Design review of the part built by this model. Coordinates are the model's own, in mm. A direction names the side the tool comes from. Give positions to 0.01 mm unless a question says otherwise; leave off trailing zeros. Order: outer loops, then holes, each group sorted by start corner. A loop starts at its lowest first (then second) coordinate and runs counter-clockwise, first axis right, second up.
```python
from build123d import *

# Parameters (mm, degrees)
PAD_DEPTH    = 1
PAD001_DEPTH = 1
SKETCH002_W  = 3.5
SKETCH002_H  = 2
PAD002_DEPTH = 10
SKETCH003_R  = 2.5
POCKET_DEPTH = 2.001
SKETCH004_R  = 0.5
HOLE_DEPTH   = 10
HOLE_TIPS_R  = 0.5


with BuildPart() as part:
    # Sketch → Pad (new body)
    with BuildSketch(Plane.XY):
        with BuildLine():
            Line((-10, 5), (10, 5))
            Line((10, 5), (10, 1.5))
            ThreePointArc((10, -1.5), (11.5, 0), (10, 1.5))
            Line((10, -1.5), (10, -5))
            Line((10, -5), (-10, -5))
            Line((-10, -5), (-10, -1.5))
            ThreePointArc((-10, 1.5), (-11.5, 0), (-10, -1.5))
            Line((-10, 1.5), (-10, 5))
        make_face()
    extrude(amount=PAD_DEPTH)

    # Sketch001 (on Face10 of Pad) → Pad001 (join)
    with BuildSketch(Plane.XY.offset(1)):
        Polygon((-9, 4), (9, 4), (9, 0.489518), (7, 0.489518), (7, -0.510482), (9, -0.510482), (9, -4), (-9, -4), (-9, -0.49649), (-7, -0.49649), (-7, 0.50351), (-9, 0.50351), align=None)
    extrude(amount=PAD001_DEPTH)

    # Sketch002 (on Face23 of Pad001) → Pad002 (join)
    with BuildSketch(Plane.XY.offset(2)):
        with Locations((7.25, -3)):
            Rectangle(SKETCH002_W, SKETCH002_H)
        with Locations((7.25, 3)):
            Rectangle(SKETCH002_W, SKETCH002_H)
        with Locations((-7.25, 3)):
            Rectangle(SKETCH002_W, SKETCH002_H)
        with Locations((-7.25, -3)):
            Rectangle(SKETCH002_W, SKETCH002_H)
    extrude(amount=PAD002_DEPTH)

    # Sketch003 (on Face23 of Pad002) → Pocket (cut, through all)
    with BuildSketch(Plane.XY.offset(2)):
        Circle(SKETCH003_R)
    extrude(amount=-POCKET_DEPTH, mode=Mode.SUBTRACT)

    # Sketch004 (on Face42 of Pocket) → Hole (cut)
    with BuildSketch(Plane.XY.offset(12)):
        with Locations((8, -3)):
            Circle(SKETCH004_R)
        with Locations((-8, 3)):
            Circle(SKETCH004_R)
        with Locations((-8, -3)):
            Circle(SKETCH004_R)
        with Locations((8, 3)):
            Circle(SKETCH004_R)
    extrude(amount=-HOLE_DEPTH, mode=Mode.SUBTRACT)

    # Hole tips → Hole tip 1 section 0
    with BuildSketch(Plane.XY.offset(2), mode=Mode.PRIVATE) as hole_tip_1_s0:
        with Locations((8, -3)):
            Circle(HOLE_TIPS_R)
    loft([hole_tip_1_s0.sketch, Vertex(8, -3, 1.69957)], mode=Mode.SUBTRACT)

    # Hole tips → Hole tip 2 section 0
    with BuildSketch(Plane.XY.offset(2), mode=Mode.PRIVATE) as hole_tip_2_s0:
        with Locations((-8, 3)):
            Circle(HOLE_TIPS_R)
    loft([hole_tip_2_s0.sketch, Vertex(-8, 3, 1.69957)], mode=Mode.SUBTRACT)

    # Hole tips → Hole tip 3 section 0
    with BuildSketch(Plane.XY.offset(2), mode=Mode.PRIVATE) as hole_tip_3_s0:
        with Locations((-8, -3)):
            Circle(HOLE_TIPS_R)
    loft([hole_tip_3_s0.sketch, Vertex(-8, -3, 1.69957)], mode=Mode.SUBTRACT)

    # Hole tips → Hole tip 4 section 0
    with BuildSketch(Plane.XY.offset(2), mode=Mode.PRIVATE) as hole_tip_4_s0:
        with Locations((8, 3)):
            Circle(HOLE_TIPS_R)
    loft([hole_tip_4_s0.sketch, Vertex(8, 3, 1.69957)], mode=Mode.SUBTRACT)


solid = part.part
```
1. Machinability: for faces 5 (the face through (-10, -3.3, 0.5)), 6 (the face through (10, -3.2, 0.5)), 7 (the face through (-7, 2, 7)), 8 (the face through (-7, 0, 1.5)), which of the approach directions +Z, -Z, +X, -X, +Y, -Y give a long, thin tool a straight path to every point of the face, cutting with its end or side? Answer none if there is none.
Recorded:
face 5: +Z, -Z, -X, -Y
face 6: +Z, -Z, +X, -Y
face 7: +Z, +X, -X
face 8: +Z, -X
2. For pin 1 (6 mm diameter, centred on y = -3, z = 3, fed in from +X); pin 2 (1.1 mm diameter, centred on y = -4, z = 0.5, fed in from -X); pin 3 (1.6 mm diameter, centred on y = -3.5, z = 7, fed in from +X); pin 4 (4 mm diameter, centred on x = 0, y = 0, fed in from -Z), all flat-tipped, find the tip position at first contact; note any pin that passes through.
Recorded:
pin 1: stops at x = 11.29
pin 2: stops at x = -10
pin 3: stops at x = 9
pin 4: passes through
3. Draft analysis for pull direction X (two halves, no side actions). For faces 1 (the face through (-10, 3.2, 0.5)), 2 (the face through (8, -0.51, 1.5)), 3 (the face through (8.074, 2.969, 1.748)), 4 (the face through (8.074, -3.031, 1.748)), state which applies: pulls with the +X half, pulls with the -X half, needs draft (parallel to the pull), parting line crosses it, or undercut.
Recorded:
face 1: pulls with the -X half
face 2: needs draft
face 3: undercut
face 4: undercut
4. Take a section at B-B (x = 4.75). State the section outline as (y, z) points, then the cut area to 3 significant figures.
Recorded:
outline: (-5, 0) - (5, 0) - (5, 1) - (4, 1) - (4, 2) - (-4, 2) - (-4, 1) - (-5, 1) - close
area: 18.0 mm2
5. Take a section at A-A (z = 3). State the section outline as (x, y) points, then the cut area to 3 significant figures.
Recorded:
outline: (-9, -4) - (-5.5, -4) - (-5.5, -2) - (-9, -2) - close; (-9, 2) - (-5.5, 2) - (-5.5, 4) - (-9, 4) - close; (5.5, -4) - (9, -4) - (9, -2) - (5.5, -2) - close; (5.5, 2) - (9, 2) - (9, 4) - (5.5, 4) - close; hole circle Ø1 at (-8, -3); hole circle Ø1 at (-8, 3); hole circle Ø1 at (8, -3); hole circle Ø1 at (8, 3)
area: 24.9 mm2
6. Take a section at C-C (y = 0). State the section outline as (x, z) points, then the cut area to 3 significant figures.
Recorded:
outline: (-11.5, 0) - (-2.5, 0) - (-2.5, 2) - (-7, 2) - (-7, 1) - (-11.5, 1) - close; (2.5, 0) - (11.5, 0) - (11.5, 1) - (7, 1) - (7, 2) - (2.5, 2) - close
area: 27.0 mm2
7. For line 1 along Y through (x, z) = (-8, 8); line 2 along Y through (x, z) = (5.75, 4.25); line 3 along Y through (x, z) = (0, 1.5), list the stretches that pass through material, from the lowest coordinate up.
Recorded:
line 1: y = -4 to -3.5, -2.5 to -2, 2 to 2.5, 3.5 to 4
line 2: y = -4 to -2, 2 to 4
line 3: y = -4 to -2.5, 2.5 to 4
8. Take a section at D-D (x = -0.25). State the section outline as (y, z) points, then the cut area to 3 significant figures.
Recorded:
outline: (-5, 0) - (-2.49, 0) - (-2.49, 2) - (-4, 2) - (-4, 1) - (-5, 1) - close; (2.49, 0) - (5, 0) - (5, 1) - (4, 1) - (4, 2) - (2.49, 2) - close
area: 8.05 mm2
